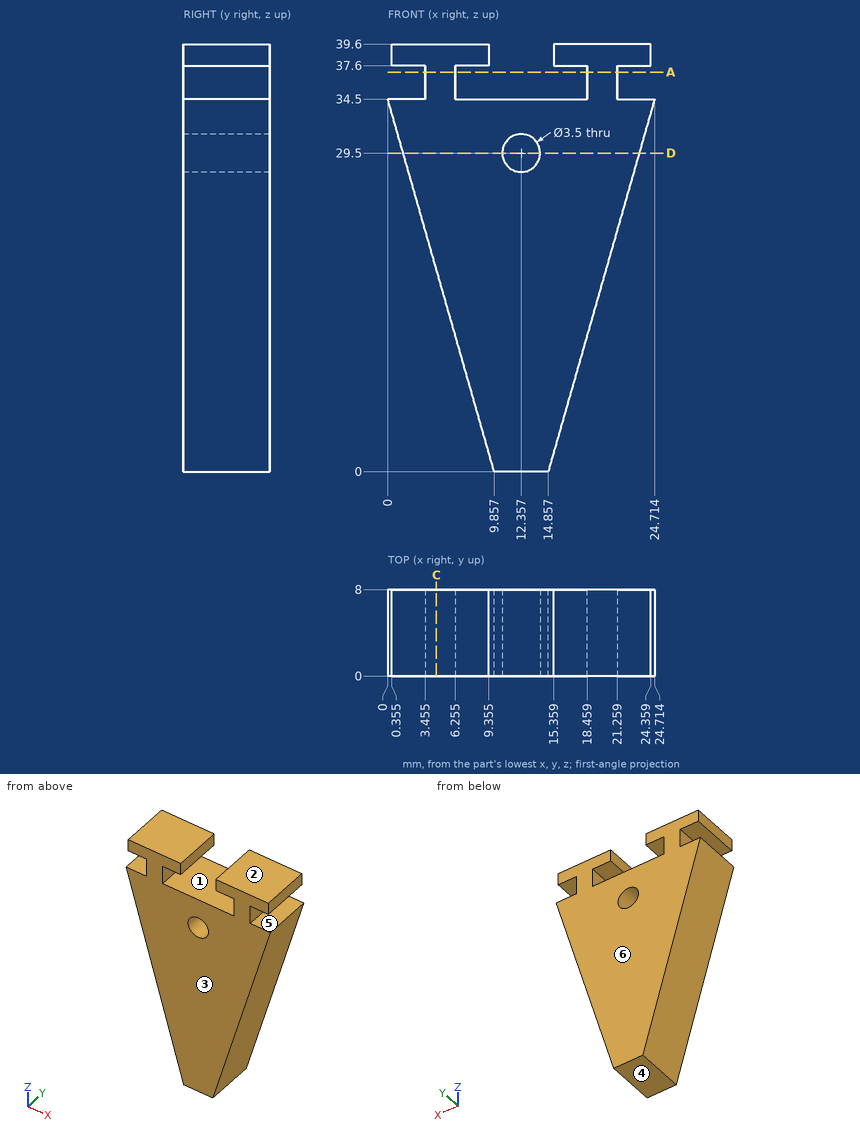
Could you check a few things on this drawing? It's one solid part, dimensions in mm from its lowest x, y, z. A direction names the side the tool comes from. Coordinates: 2 decimals unless noted, no trailing zeros. Order: outer loops, then holes, each group sorted by start corner. A loop starts at its lowest first (then second) coordinate and runs counter-clockwise, first axis right, second up. Notation, with made-up numbers: M 80.25,-26 L 93.25,-26 A11 ccw 93.25,-9 Z; hole C -37.5,34.25 d4. An arc over 180 degrees is marked long. Use one line per item in the form item = value. Start each with the question number.
1. Suppose I cut it at A-A on z = 37. Write out the boundary of the cut face in (x, y) (1 decimal), then the cut area to 3 significant figures.
2. On a 3-axis mill with a long thin cutter (end or side, diameter ignored), from which of +Z, -Z, +X, -X, +Y, -Y can I reach the whole of each face in a straight line? I mean the marked faces 5 and 6. Say none if no direction works.
3. Please list where these lines run through material, in increasing order: line 1 (Z direction, x = 12.5, y = 4.75) (1 decimal); line 2 (X direction, y = 3.75, z = 38.5) (1 decimal); line 3 (X direction, y = 3, z = 30) (1 decimal).
4. For pin 1 (4 mm diameter, centred on x = 14.5, y = 3.5, fed in from +Z); pin 2 (1.6 mm diameter, centred on y = 4.5, z = 36.5, fed in from +X); pin 3 (2 mm diameter, centred on y = 2.5, z = 39, fed in from -X) (1 decimal); pin 4 (1 mm diameter, centred on y = 2, z = 23, fed in from -X), each with a flat end and sliding along its axis, tell me the tip position at first contact or that it passes through.
5. Suppose I cut it at C-C on x = 4.5. Write out the boundary of the cut face in (y, z).
6. We'd pull the mould along Z, two halves only. Please class the marked faces 1, 2, 3 and 4: +Z half, -Z half, draft (parallel to the pull), parting line (faces both ways), or undercut.
7. Suppose I cut it at D-D on z = 29.5. Write out the boundary of the cut face in (x, y) (1 decimal).
Geometry says:
q1.outline = M 3.5,0 L 6.3,0 L 6.3,8 L 3.5,8 Z; M 18.5,0 L 21.3,0 L 21.3,8 L 18.5,8 Z
q1.area = 44.8 mm^2
q2.face_5 = +X, +Y, -Y
q2.face_6 = +Z, -Z, +X, -X, +Y
q3.line_1 = 0 to 27.8, 31.2 to 34.5
q3.line_2 = 0.4 to 9.4, 15.4 to 24.4
q3.line_3 = 1.3 to 10.7, 14 to 23.4
q4.pin_1 = 39.6
q4.pin_2 = 21.26
q4.pin_3 = 0.4
q4.pin_4 = 3.14
q5.outline = M 0,18.75 L 8,18.75 L 8,39.6 L 0,39.6 Z
q6.face_1 = undercut
q6.face_2 = +Z half
q6.face_3 = draft
q6.face_4 = -Z half
q7.outline = M 1.4,0 L 10.6,0 L 10.6,8 L 1.4,8 Z; M 14.1,0 L 23.3,0 L 23.3,8 L 14.1,8 Z
